```python
from build123d import *

# Parameters (mm, degrees)
F1_DEPTH = 1.6
F0_W     = 15
F0_H     = 12
F2_DEPTH = 4.5
F3_W     = 2.5
F3_H     = 16
F4_DEPTH = 2.4


with BuildPart() as f1:
    # F0 (on Top) → F1 (new body)
    with BuildSketch(Plane.XY):
        Polygon((-15, -0.567309), (-48, -0.567309), (-48, -17.567309), (-15, -17.567309), (-15, -14.936926), (-15, -2.936926), align=None)
    extrude(amount=F1_DEPTH)

    # F0 (on Top) → F2 (join)
    with BuildSketch(Plane.XY):
        with Locations((-7.5, -8.936926)):
            Rectangle(F0_W, F0_H)
    extrude(amount=F2_DEPTH)

    # F3 (on face) → F4 (join)
    with BuildSketch(Plane.XY.offset(1.6)):
        with Locations((-46.25, -9.064941)):
            Rectangle(F3_W, F3_H)
    extrude(amount=F4_DEPTH)


solid = f1.part
```
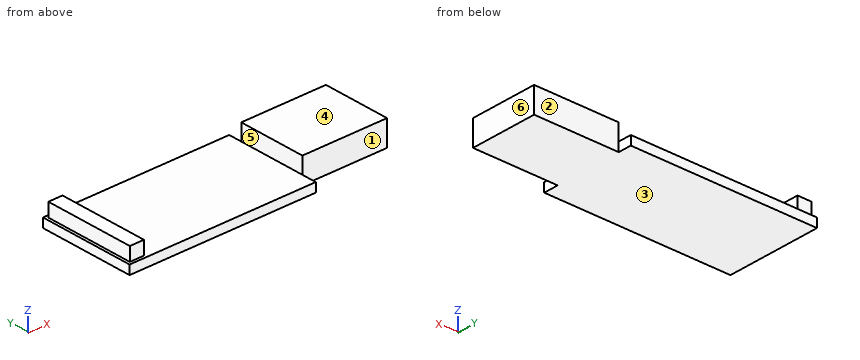
Verification items for the finished model (mm, model axes). Face numbers are marked on the shaded views. A direction names the side the tool comes from. Coordinates: 2 decimals unless noted, no trailing zeros. Write each loop counter-clockwise with the first axis right and the second up, starting at its lowest first coordinate (ties: lowest second). Pieces come first, ordered by that corner, then holes. Notation, with made-up numbers: (44, -5.75) - (90, -5.75) arc R6 ccw to (90, 3.25) - close; hole circle Ø1 at (85, -8). An arc over 180 degrees is marked (long way). Write item = value, one per line.
Q1. Cross-section at C-C (z = 0.5). Enter the section's corners in (x, y).
Answer:
outline = (-48, -17.57) - (-15, -17.57) - (-15, -14.94) - (0, -14.94) - (0, -2.94) - (-15, -2.94) - (-15, -0.57) - (-48, -0.57) - close
Q2. Cross-section at B-B (y = -15.5). Enter the section's corners in (x, z).
Answer:
outline = (-48, 0) - (-15, 0) - (-15, 1.6) - (-45, 1.6) - (-45, 4) - (-47.5, 4) - (-47.5, 1.6) - (-48, 1.6) - close
Q3. Cross-section at D-D (x = -13). Enter the section's corners in (y, z), plus the area to 3 significant figures.
Answer:
outline = (-14.94, 0) - (-2.94, 0) - (-2.94, 4.5) - (-14.94, 4.5) - close
area = 54.0 mm²
Q4. Go/stop test with flat-tipped pins: pin 1 Ø8.5 at (x, y) = (-31.5, -11) entering from +Z; pin 2 Ø0.9 at (y, z) = (-10.5, 3) entering from -X; pin 3 Ø6 at (x, y) = (-42.5, -9.5) entering from +Z. Record where each tip stops, or that it passes through.
Answer:
pin_1 = 1.6
pin_2 = -47.5
pin_3 = 4
Q5. Cross-section at A-A (z = 2.65). Enter the section's corners in (x, y), plus the area to 3 significant figures.
Answer:
outline = (-47.5, -17.06) - (-45, -17.06) - (-45, -1.06) - (-47.5, -1.06) - close; (-15, -14.94) - (0, -14.94) - (0, -2.94) - (-15, -2.94) - close
area = 220 mm²
Q6. Material ranges on L1, parallel to X at y = -9, z = 3.65; L2, parallel to Z at x = -29, y = -14.75; L3, parallel to Y at x = -11.5, z = 1.45, recorded low to high. Write a range as from..to.
Answer:
L1 = -47.5..-45, -15..0
L2 = 0..1.6
L3 = -14.94..-2.94
Q7. Mould release check, pull along X, two halves, no side actions. Record for the marked faces 4, 5 and 6: released by +X, released by -X, zero draft, split by the parting line, or undercut.
Answer:
face_4 = zero draft
face_5 = undercut
face_6 = released by +X
Q8. Access from +Z, -Z, +X, -X, +Y, -Y to the whole of each face (thin tool, end or side, straight path). Record for the marked faces 1, 2 and 3.
Answer:
face_1 = +Z, -Z, +X, -Y
face_2 = +Z, -Z, +X, +Y
face_3 = -Z, +X, -X, +Y, -Y
